```python
from build123d import *

# Parameters (mm, degrees)
SKETCH1_W                        = 19.05
SKETCH1_H                        = 88.9
BOSS_EXTRUDE1_DEPTH              = 6.35
F_1_4_20_TAPPED_HOLE1_AT_2_COUNT = 2
F_1_4_20_TAPPED_HOLE1_AT_2_PITCH = 28.575
F_1_4_20_TAPPED_HOLE1_AT_3_COUNT = 2
F_1_4_20_TAPPED_HOLE1_AT_3_PITCH = 57.15


with BuildPart() as part:
    # Sketch1 → Boss-Extrude1 (new body)
    with BuildSketch(Plane(origin=(0, 0, 0), x_dir=(1, 0, 0), z_dir=(0, 1, 0))):
        with Locations((-9.525, 44.45)):
            Rectangle(SKETCH1_W, SKETCH1_H)
    extrude(amount=BOSS_EXTRUDE1_DEPTH)

    # Sketch3 → 1/4-20 Tapped Hole1 (revolve, cut)
    with BuildSketch(Plane(origin=(-12.7, 6.35, -15.875), x_dir=(0, 0, 1), z_dir=(1, 0, 0))):
        Polygon((0, 0), (0, 6.35), (2.5527, 6.35), (2.5527, 4.368293953), (6.35, 0), align=None)
    f_1_4_20_tapped_hole1 = revolve(axis=Axis((-12.7, 12.7, -15.875), (0, -1, 0)), mode=Mode.SUBTRACT)

    # 1/4-20 Tapped Hole1 at 2: 1/4-20 Tapped Hole1 ×2
    with Locations(*[(0, 0, -i * F_1_4_20_TAPPED_HOLE1_AT_2_PITCH) for i in range(1, F_1_4_20_TAPPED_HOLE1_AT_2_COUNT)]):
        add(f_1_4_20_tapped_hole1, mode=Mode.SUBTRACT)

    # 1/4-20 Tapped Hole1 at 3: 1/4-20 Tapped Hole1 ×2
    with Locations(*[(0, 0, -i * F_1_4_20_TAPPED_HOLE1_AT_3_PITCH) for i in range(1, F_1_4_20_TAPPED_HOLE1_AT_3_COUNT)]):
        add(f_1_4_20_tapped_hole1, mode=Mode.SUBTRACT)


solid = part.part
```
Source: CAD feature listing. Evaluate the final solid. Frame: model axes, mm. Round coordinates to 2 decimals unless told otherwise and drop trailing zeros. Loops run counter-clockwise (first coordinate to the right, second up) from the corner with the lowest first, then second, coordinate; pieces in that order, holes last. Notation, with made-up numbers: M -16.5,76 L -1.5,76 A23 cw -1.5,102 Z; hole C 83.25,-29 d3. An arc over 180 degrees is marked long. Put each result on its own line as item: value.
(1) Section B-B, the plane y = 3.5. Return loops of the section in (x, z) (3 decimals).
Solutions:
outline: M -19.05,-88.9 L 0,-88.9 L 0,0 L -19.05,0 Z; hole C -12.7,-73.025 d7.745; hole C -12.7,-44.45 d7.745; hole C -12.7,-15.875 d7.745
(2) Pull-direction query (Z, two-part tool) for faces 1 (the face through (-10, 3, -88.9)), 2 (the face through (-11.63, 2.25, -70.45)), 3 (the face through (0, 3, -44)), 4 (the face through (-10.435, 1.005, -14.697)); classes: released by +Z, released by -Z, zero draft, split by the parting line, or undercut.
Solutions:
face 1: released by -Z
face 2: undercut
face 3: zero draft
face 4: undercut
(3) Section A-A, the plane x = -12.7. Return loops of the section in (y, z) (3 decimals).
Solutions:
outline: M 0,-88.9 L 6.35,-88.9 L 6.35,-79.375 L 1.982,-75.578 L 0,-75.578 Z; M 0,-70.472 L 1.982,-70.472 L 6.35,-66.675 L 6.35,-50.8 L 1.982,-47.003 L 0,-47.003 Z; M 0,-41.897 L 1.982,-41.897 L 6.35,-38.1 L 6.35,-22.225 L 1.982,-18.428 L 0,-18.428 Z; M 0,-13.322 L 1.982,-13.322 L 6.35,-9.525 L 6.35,0 L 0,0 Z
(4) Ray query, line 1 (Z direction, x = -12.7, y = 1); line 2 (X direction, y = 1.35, z = -44.45); line 3 (Z direction, x = -17, y = 6.25). Return the intervals inside material, ascending. Write a range as [from, to].
Solutions:
line 1: [-88.9, -75.58], [-70.47, -47], [-41.9, -18.43], [-13.32, 0]
line 2: [-19.05, -15.25], [-10.15, 0]
line 3: [-88.9, -77.58], [-68.47, -49], [-39.9, -20.43], [-11.32, 0]
(5) First-contact query: pin 1 (8 mm diameter, centred on x = -12.7, z = -15.875, fed in from +Y). Flat tip, straight axial feed; report the tip coordinate or a pass-through.
Solutions:
pin 1: y = 3.65
